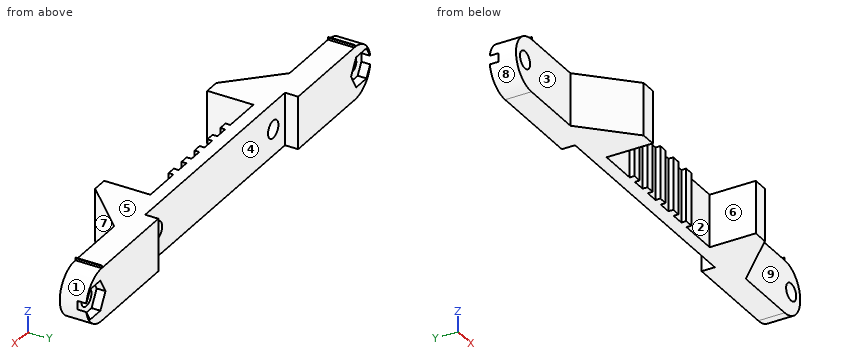
from build123d import *

# Parameters (mm, degrees)
SKETCH1_R                 = 1.95
BOSS_EXTRUDE1_DEPTH       = 3
SKETCH4_W                 = 3.5
SKETCH4_H                 = 12
BOSS_EXTRUDE3_DEPTH       = 10.5
SKETCH5_W                 = 2
SKETCH5_H                 = 12
BOSS_EXTRUDE4_DEPTH       = 1.1
SKETCH6_W                 = 0.2
SKETCH6_H                 = 3
BOSS_EXTRUDE5_DEPTH       = 0.5
CHAMFER1_SIZE             = 10.5
BOSS_EXTRUDE6_OUTLINE_R   = 1.95
BOSS_EXTRUDE6_OUTLINE_R_2 = 1.45
BOSS_EXTRUDE6_DEPTH       = 3
CUT_EXTRUDE1_START        = -2
SKETCH11_R                = 1.45
CUT_EXTRUDE1_DEPTH        = 2
SKETCH13_R                = 2
CUT_EXTRUDE2_DEPTH        = 8


# Read off the part's stored shape, not the designer's step: Boss-Extrude6
with BuildPart() as part:
    # Sketch1 → Boss-Extrude1 (new body)
    with BuildSketch(Plane(origin=(0, 0, 0), x_dir=(1, 0, 0), z_dir=(0, 1, 0))):
        with BuildLine():
            Line((-49, 6), (49, 6))
            ThreePointArc((49, 6), (55, 0), (49, -6))
            Line((49, -6), (-49, -6))
            ThreePointArc((-49, -6), (-55, 0), (-49, 6))
        make_face()
        with Locations(Location((-51.5, 0, 0), (0, 0, 270))):
            Circle(SKETCH1_R, mode=Mode.SUBTRACT)
        with Locations(Location((51.5, 0, 0), (0, 0, 270))):
            Circle(SKETCH1_R, mode=Mode.SUBTRACT)
    extrude(amount=BOSS_EXTRUDE1_DEPTH)

    # Sketch4 → Boss-Extrude3 (add)
    with BuildSketch(Plane.XZ):
        with Locations((-21.690023983, 0)):
            Rectangle(SKETCH4_W, SKETCH4_H)
        with Locations((21.690023983, 0)):
            Rectangle(SKETCH4_W, SKETCH4_H)
    extrude(amount=BOSS_EXTRUDE3_DEPTH)

    # Sketch5 → Boss-Extrude4 (add)
    with BuildSketch(Plane.XZ):
        with Locations((5, 0)):
            Rectangle(SKETCH5_W, SKETCH5_H)
        Rectangle(SKETCH5_W, SKETCH5_H)
        with Locations((10, 0)):
            Rectangle(SKETCH5_W, SKETCH5_H)
        with Locations((-5, 0)):
            Rectangle(SKETCH5_W, SKETCH5_H)
        with Locations((-10, 0)):
            Rectangle(SKETCH5_W, SKETCH5_H)
    extrude(amount=BOSS_EXTRUDE4_DEPTH)

    # Sketch6 → Boss-Extrude5 (add)
    with BuildSketch(Plane.XY.offset(6)):
        with Locations((48.9, 1.5)):
            Rectangle(SKETCH6_W, SKETCH6_H)
        with Locations((-48.9, 1.5)):
            Rectangle(SKETCH6_W, SKETCH6_H)
    extrude(amount=BOSS_EXTRUDE5_DEPTH)

    # Chamfer1
    chamfer1_edges = [part.edges().sort_by_distance(p)[0] for p in [
        (23.440023983, 0, 0),
        (-23.440023983, 0, 0),
    ]]
    chamfer(chamfer1_edges, length=CHAMFER1_SIZE - 0.0001)  # a hair under: the kernel refuses the full size

    # Boss-Extrude6 outline → Boss-Extrude6 (add)
    # profile 1 of 2: a face of its own
    with BuildSketch(Plane(origin=(0, 3, 0), x_dir=(1, 0, 0), z_dir=(0, 1, 0))):
        with BuildLine():
            Line((27.05, -6), (48.8, -6))
            Line((48.8, -6), (48.8, -6.5))
            Line((48.8, -6.5), (49, -6.5))
            Line((49, -6.5), (49, -6))
            ThreePointArc((49, -6), (55, 0), (49, 6))
            Line((49, 6), (27.05, 6))
            Line((27.05, 6), (27.05, -6))
        make_face()
        with Locations((51.5, 0)):
            Circle(BOSS_EXTRUDE6_OUTLINE_R, mode=Mode.SUBTRACT)
    # profile 2 of 2: a face of its own
    with BuildSketch(Plane(origin=(0, 3, 0), x_dir=(1, 0, 0), z_dir=(0, 1, 0))):
        with BuildLine():
            Line((-48.8, -6), (-27.05, -6))
            Line((-27.05, -6), (-27.05, 6))
            Line((-27.05, 6), (-49, 6))
            ThreePointArc((-49, 6), (-55, 0), (-49, -6))
            Line((-49, -6), (-49, -6.5))
            Line((-49, -6.5), (-48.8, -6.5))
            Line((-48.8, -6.5), (-48.8, -6))
        make_face()
        with Locations((-51.5, 0)):
            Circle(BOSS_EXTRUDE6_OUTLINE_R_2, mode=Mode.SUBTRACT)
    extrude(amount=BOSS_EXTRUDE6_DEPTH)

    # Sketch11 → Cut-Extrude1 (cut)
    # profile 1 of 2: a face of its own
    with BuildSketch(Plane(origin=(0, 6, 0), x_dir=(1, 0, 0), z_dir=(0, 1, 0)).offset(CUT_EXTRUDE1_START)):
        Polygon((53.491858429, 3.45), (55.483716857, 0), (53.491858429, -3.45), (49.508141571, -3.45), (47.516283143, 0), (49.508141571, 3.45), align=None)
    # profile 2 of 2: a face of its own
    with BuildSketch(Plane(origin=(0, 6, 0), x_dir=(1, 0, 0), z_dir=(0, 1, 0)).offset(CUT_EXTRUDE1_START)):
        Polygon((-47.516283143, 0), (-49.508141571, 3.45), (-53.491858429, 3.45), (-55.483716857, 0), (-53.491858429, -3.45), (-49.508141571, -3.45), align=None)
        with Locations(Location((-51.5, 0, 0), (0, 0, 270))):
            Circle(SKETCH11_R, mode=Mode.SUBTRACT)
    extrude(amount=CUT_EXTRUDE1_DEPTH, mode=Mode.SUBTRACT)

    # Sketch13 → Cut-Extrude2 (cut)
    with BuildSketch(Plane(origin=(0, 3, 0), x_dir=(1, 0, 0), z_dir=(0, 1, 0))):
        with Locations(Location((22.5, 0, 0), (0, 0, 270))):
            Circle(SKETCH13_R)
        with Locations(Location((-22.5, 0, 0), (0, 0, 270))):
            Circle(SKETCH13_R)
    extrude(amount=-CUT_EXTRUDE2_DEPTH, mode=Mode.SUBTRACT)


solid = part.part
Here's how the part is built. I have some questions about the finished solid (model axes, mm). Face numbers are marked on the shaded views. A direction names the side the tool comes from. Round coordinates to 2 decimals unless told otherwise and drop trailing zeros. Write each loop counter-clockwise with the first axis right and the second up, starting at its lowest first coordinate (ties: lowest second). Pieces come first, ordered by that corner, then holes.
1. Suppose I cut it at A-A (y = -3.25). List the corners of the cut face in (x, z) for me, and give its area (3 significant figures).
2. I need wall thicknesses on L1, parallel to X at y = 0.85, z = 0; L2, parallel to X at y = -1.5, z = -1; L3, parallel to Y at x = 7, z = 1.25. Which ranges of each line are inside material? Lowest first, please.
3. Suppose I cut it at C-C (y = -7.25). List the corners of the cut face in (x, z) for me, and give its area (3 significant figures).
4. Suppose I cut it at D-D (x = 13). List the corners of the cut face in (y, z) for me, and give its area (3 significant figures).
5. Suppose I cut it at B-B (x = -51.5). List the corners of the cut face in (y, z) for me.
6. Will these pins go through, and if not, where does the flat tip stop? pin 1 Ø0.9 at (y, z) = (-0.5, 1.5) entering from +X; pin 2 Ø6 at (x, z) = (5.5, -4.5) entering from +Y; pin 3 Ø1 at (x, z) = (0, -1) entering from -Y.
7. For the marked faces 1, 2, 3, 4 and 5, which set-ups out of +Z, -Z, +X, -X, +Y, -Y let a thin tool reach every point of the face, with its end or its side?
8. If we mould it in two halves opening along X, with no side actions, what happens to the marked faces 6, 7, 8 and 9? For each: released by +X, released by -X, zero draft, split by the parting line, or undercut.
Answer sheet:
1. outline: (-30.69, -6) - (-19.94, -6) - (-19.94, 6) - (-30.69, 6) - close; (19.94, -6) - (30.69, -6) - (30.69, 6) - (19.94, 6) - close; hole circle Ø4 at (-22.5, 0); hole circle Ø4 at (22.5, 0)
1. area: 233 mm2
2. L1: x = -55 to -53.45, -49.55 to -24.5, -20.5 to 20.5, 24.5 to 49.55, 53.45 to 55
2. L2: x = -32.44 to -24.23, -20.77 to -19.94, 19.94 to 20.77, 24.23 to 32.44
2. L3: y = 0 to 3
3. outline: (-26.69, -6) - (-19.94, -6) - (-19.94, 6) - (-26.69, 6) - close; (19.94, -6) - (26.69, -6) - (26.69, 6) - (19.94, 6) - close
3. area: 162 mm2
4. outline: (0, -6) - (3, -6) - (3, 6) - (0, 6) - close
4. area: 36.0 mm2
5. outline: (0, -5.45) - (6, -5.45) - (6, -3.45) - (4, -3.45) - (4, -1.45) - (3, -1.45) - (3, -1.95) - (0, -1.95) - close; (0, 1.95) - (3, 1.95) - (3, 1.45) - (4, 1.45) - (4, 3.45) - (6, 3.45) - (6, 5.45) - (0, 5.45) - close
6. pin 1: stops at x = 33.89
6. pin 2: stops at y = 3
6. pin 3: stops at y = -1.1
7. face 1: +X, +Y, -Y
7. face 2: +Z, -Z, -Y
7. face 3: +Z, -Z, -X, -Y
7. face 4: +Z, -Z, +Y
7. face 5: +Z, +Y, -Y
8. face 6: undercut
8. face 7: released by +X
8. face 8: released by -X
8. face 9: zero draft
